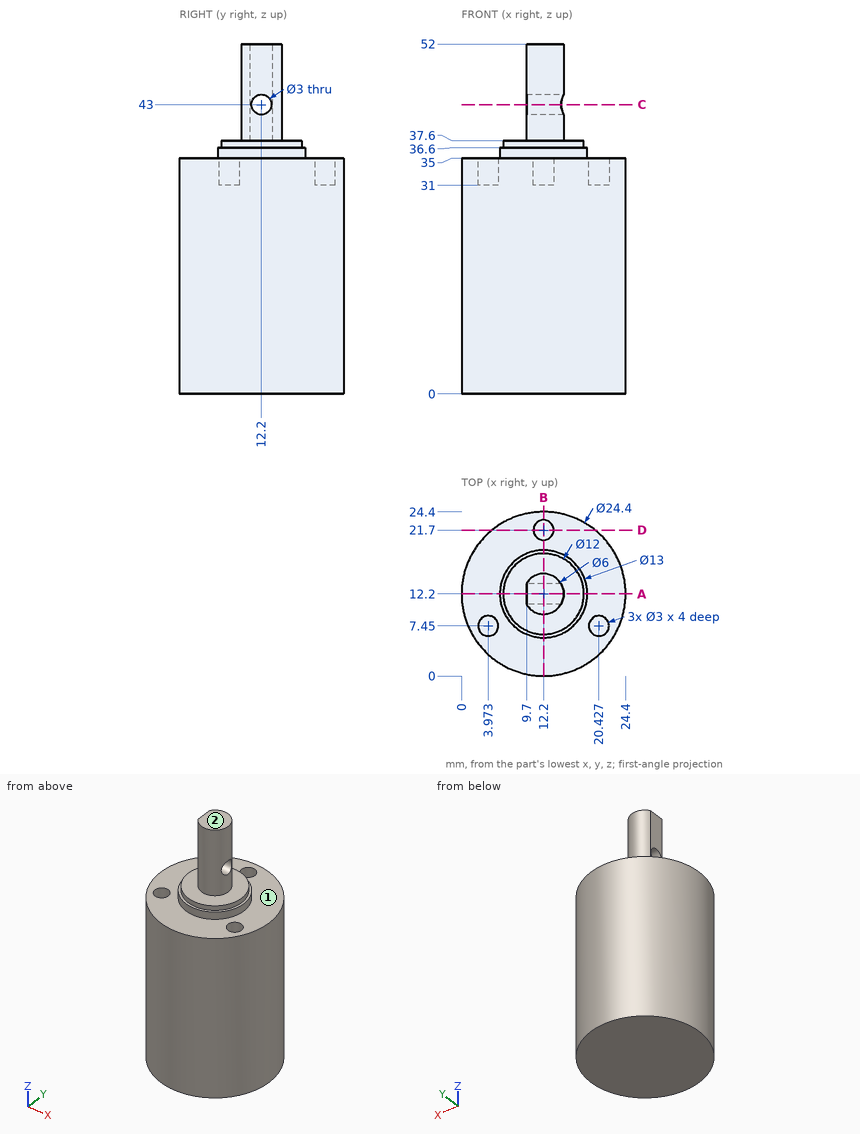
Verification items for this drawing (mm, ordinates from the low corner). A direction names the side the tool comes from. Coordinates: 2 decimals unless noted, no trailing zeros. Write each loop counter-clockwise with the first axis right and the second up, starting at its lowest first coordinate (ties: lowest second). Pieces come first, ordered by that corner, then holes. Notation, with made-up numbers: M 73,79.25 L 123,79.25 A26 ccw 123,96.25 Z; hole C 51,71 d7. An arc over 180 degrees is marked long. Answer as a JSON object with one key per item and string values. Group by question number.
(1) Tool access check on the marked faces 1 and 2. Record the directions out of +Z, -Z, +X, -X, +Y, -Y that give a thin tool (end or side, any length) a straight path to the whole face; none if there is none.
(2) Gauge pin test, flat ends, axial feed: pin 1 (4 mm diameter, centred on y = 12.2, z = 43, fed in from -X); pin 2 (3 mm diameter, centred on x = 16.5, z = 27.5, fed in from +Y); pin 3 (1.5 mm diameter, centred on x = 4, y = 8, fed in from +Z). Record the tip position at first contact, or that the pin passes through.
(3) Cross-section at A-A, the plane y = 12.2. Record the cut outline in (x, z).
(4) Cross-section at C-C, the plane z = 43. Record the cut outline in (x, y).
(5) Material ranges on line 1 (Z direction, x = 14, y = 12); line 2 (Z direction, x = 4.75, y = 20.25); line 3 (Z direction, x = 6.5, y = 9.5), recorded low to high.
(6) Cross-section at B-B, the plane x = 12.2. Record the cut outline in (y, z), and give its area (3 significant figures).
(7) Cross-section at D-D, the plane y = 21.7. Record the cut outline in (x, z).
Reply:
{
 "1": {"face 1": "+Z", "face 2": "+Z, +X, -X, +Y, -Y"},
 "2": {"pin 1": "x = 9.7", "pin 2": "y = 24.07", "pin 3": "z = 31"},
 "3": {"outline": "M 0,0 L 24.4,0 L 24.4,35 L 18.7,35 L 18.7,36.6 L 18.2,36.6 L 18.2,37.6 L 15.2,37.6 L 15.2,41.5 L 9.7,41.5 L 9.7,37.6 L 6.2,37.6 L 6.2,36.6 L 5.7,36.6 L 5.7,35 L 0,35 Z; M 9.7,44.5 L 15.2,44.5 L 15.2,52 L 9.7,52 Z"},
 "4": {"outline": "M 9.7,10.54 A3 ccw 14.8,10.7 L 9.7,10.7 Z; M 9.7,13.7 L 14.8,13.7 A3 ccw 9.7,13.86 Z"},
 "5": {"line 1": "0 to 41.51, 44.49 to 52", "line 2": "0 to 35", "line 3": "0 to 36.6"},
 "6": {"outline": "M 0,0 L 24.4,0 L 24.4,35 L 23.2,35 L 23.2,31 L 20.2,31 L 20.2,35 L 18.7,35 L 18.7,36.6 L 18.2,36.6 L 18.2,37.6 L 15.2,37.6 L 15.2,52 L 9.2,52 L 9.2,37.6 L 6.2,37.6 L 6.2,36.6 L 5.7,36.6 L 5.7,35 L 0,35 Z; hole C 12.2,43 d3", "area": "954 mm²"},
 "7": {"outline": "M 4.55,0 L 19.85,0 L 19.85,35 L 13.7,35 L 13.7,31 L 10.7,31 L 10.7,35 L 4.55,35 Z"}
}
